Could you check a few things on this model? Use its own coordinates, in mm. A direction names the side the tool comes from. Round coordinates to 2 decimals unless told otherwise and drop trailing zeros. Loops run counter-clockwise (first coordinate to the right, second up) from the corner with the lowest first, then second, coordinate; pieces in that order, holes last. Notation, with made-up numbers: (16.5, 30.25) -> (29.5, 30.25) arc R24 ccw to (29.5, 54.25) -> close; hole circle Ø11 at (50.25, 44.5). An arc over 180 degrees is marked (long way). Use CSV: the item, a comma, the result in double quotes. Start each with the question number.
```python
from build123d import *

# Parameters (mm, degrees)
SKETCH1_R           = 40
SKETCH1_R_2         = 4
SKETCH1_R_3         = 2.6
BOSS_EXTRUDE1_DEPTH = 10
CUT_EXTRUDE1_START  = -11
CUT_EXTRUDE1_DEPTH  = 12
CIRPATTERN1_COUNT   = 10


with BuildPart() as part:
    # Sketch1 → Boss-Extrude1 (new body)
    with BuildSketch(Plane.XY):
        Circle(SKETCH1_R)
        Circle(SKETCH1_R_2, mode=Mode.SUBTRACT)
        with Locations((-23.75, 0)):
            Circle(SKETCH1_R_3, mode=Mode.SUBTRACT)
        with Locations((-11.875, 20.56810334)):
            Circle(SKETCH1_R_3, mode=Mode.SUBTRACT)
        with Locations((11.875, 20.56810334)):
            Circle(SKETCH1_R_3, mode=Mode.SUBTRACT)
        with Locations((23.75, 0)):
            Circle(SKETCH1_R_3, mode=Mode.SUBTRACT)
        with Locations((11.875, -20.56810334)):
            Circle(SKETCH1_R_3, mode=Mode.SUBTRACT)
        with Locations((-11.875, -20.56810334)):
            Circle(SKETCH1_R_3, mode=Mode.SUBTRACT)
    extrude(amount=BOSS_EXTRUDE1_DEPTH)

    # Sketch3 → Cut-Extrude1 (cut)
    with BuildSketch(Plane.XY.offset(10).offset(CUT_EXTRUDE1_START)):
        Polygon((47.070941398, 224.331398897), (-2.338845452, 39.931563981), (-5, 30), (5, 30), (2.338845452, 39.931563981), (-47.070941398, 224.331398897), (-47.070941398, -157.478114623), (47.070941398, -157.478114623), align=None)
    cut_extrude1 = extrude(amount=CUT_EXTRUDE1_DEPTH, mode=Mode.SUBTRACT)

    # CirPattern1: Cut-Extrude1 ×10 about axis
    cirpattern1_axis = Axis((0, 0, 10), (0, 0, 1))
    for i in range(1, CIRPATTERN1_COUNT):
        add(cut_extrude1.rotate(cirpattern1_axis, i * 360 / CIRPATTERN1_COUNT), mode=Mode.SUBTRACT)


solid = part.part
```
1. Suppose I cut it at C-C (y = -26). List the corners of the cut face in (x, z) for me, then the cut area to 3 significant figures.
2. If I drill on L1, parallel to Y at x = 14, z = 6.5; L2, parallel to X at y = 25, z = 3.5; L3, parallel to X at y = 27, z = 4.25, over which ranges is the centre line in solid material (lowest first)?
3. For faces 4 (the face through (0, -30, 5)), 5 (the face through (-23.495, -26.064, 4.93)), 6 (the face through (-23.547, 26.198, 4.93)), which set-ups out of +Z, -Z, +X, -X, +Y, -Y let a thin tool reach every point of the face, with its end or its side?
4. We'd pull the mould along Y, two halves only. Please class faces 1 (the face through (12.497, 37.998, 4.93)), 2 (the face through (32, -24, 5)), 3 (the face through (17.69, -24.23, 4.93)): pulls with the +Y half, pulls with the -Y half, needs draft (parallel to the pull), parting line crosses it, or undercut.
5. Suppose I cut it at D-D (x = -23.75). List the corners of the cut face in (y, z) for me.
6. Will these pins go through, and if not, where does the flat tip stop? pin 1 (4.5 mm diameter, centred on x = 23.75, y = 0, fed in from -Z); pin 2 (1.5 mm diameter, centred on x = -30.5, z = 5, fed in from +Y); pin 3 (6 mm diameter, centred on y = -3.5, z = 8, fed in from -X); pin 4 (2 mm diameter, centred on x = -26.5, z = 5, fed in from +Y).
7. Suppose I cut it at B-B (x = 0). List the corners of the cut face in (y, z) for me.
8. Suppose I cut it at A-A (y = 0). List the corners of the cut face in (x, z) for me.
Geometry check:
1,outline,"(-30.4, 0) -> (-23.47, 0) -> (-23.47, 10) -> (-30.4, 10) -> close; (-15.25, 0) -> (15.25, 0) -> (15.25, 10) -> (-15.25, 10) -> close; (23.47, 0) -> (30.4, 0) -> (30.4, 10) -> (23.47, 10) -> close"
1,area,"444 mm²"
2,L1,"y = -37.47 to -27.54, -26.91 to -22.07, -19.07 to 19.07, 22.07 to 26.91, 27.54 to 37.47"
2,L2,"x = -31.22 to -23.09, -16.63 to 16.63, 23.09 to 31.22"
2,L3,"x = -29.51 to -23.85, -13.88 to 13.88, 23.85 to 29.51"
3,face 4,"+Z, -Z"
3,face 5,"+Z, -Z, -Y"
3,face 6,"+Z, -Z, +Y"
4,face 1,"pulls with the +Y half"
4,face 2,"pulls with the -Y half"
4,face 3,"undercut"
5,outline,"(-26.73, 0) -> (-2.6, 0) -> (-2.6, 10) -> (-26.73, 10) -> close; (2.6, 0) -> (26.73, 0) -> (26.73, 10) -> (2.6, 10) -> close"
6,pin 1,"passes through"
6,pin 2,"stops at y = 26.74"
6,pin 3,"stops at x = -40"
6,pin 4,"stops at y = 30.82"
7,outline,"(-30, 0) -> (-4, 0) -> (-4, 10) -> (-30, 10) -> close; (4, 0) -> (30, 0) -> (30, 10) -> (4, 10) -> close"
8,outline,"(-40, 0) -> (-26.35, 0) -> (-26.35, 10) -> (-40, 10) -> close; (-21.15, 0) -> (-4, 0) -> (-4, 10) -> (-21.15, 10) -> close; (4, 0) -> (21.15, 0) -> (21.15, 10) -> (4, 10) -> close; (26.35, 0) -> (40, 0) -> (40, 10) -> (26.35, 10) -> close"
